Design review of the part built by this model. Coordinates are the model's own, in mm. Coordinates: 2 decimals unless noted, no trailing zeros. Loops run counter-clockwise (first coordinate to the right, second up) from the corner with the lowest first, then second, coordinate; pieces in that order, holes last. Notation, with made-up numbers: (44.5, 56.25) -> (74.5, 56.25) arc R29 ccw to (74.5, 90.25) -> close; hole circle Ø11 at (4.5, 74.25). An arc over 180 degrees is marked (long way). Answer in a Markdown table with one row per item.
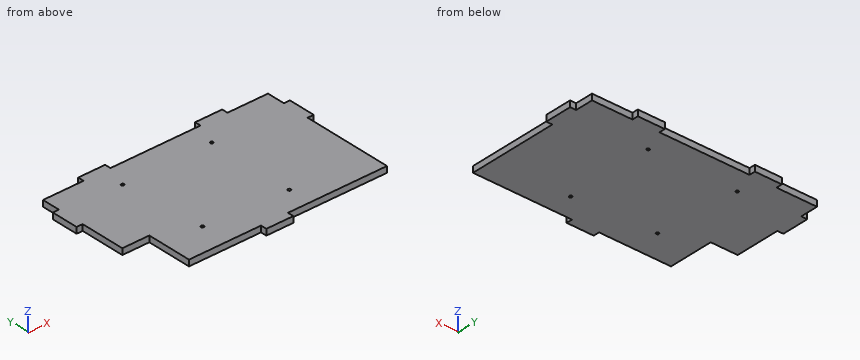
Autodesk Inventor part; units mm, degrees
ref_plane "YZ Plane" through (0, 0, 0) normal (1, 0, 0) x (0, 1, 0)
ref_plane "XZ Plane" through (0, 0, 0) normal (0, 1, 0) x (-1, 0, 0)
ref_plane "XY Plane" through (0, 0, 0) normal (0, 0, 1) x (1, 0, 0)
sketch "Sketch1" plane through (0, 0, 0) normal (0, 0, 1) x (1, 0, 0)
  line L0 (0, 0) -> (250, 0)
  line L1 (250, 0) -> (250, 150)
  line L2 (250, 150) -> (0, 150)
  line L3 (0, 150) -> (0, 0)
  dimension "d0" = 150
  dimension "d1" = 250
extrude "Extrusion1" add sketch "Sketch1" along normal blind 6.731
sketch "Sketch2" plane through (0, 0, 6.731) normal (0, 0, 1) x (1, 0, 0)
  line L0 (0, 0) -> (250, 0)
  line L1 (250, 0) -> (250, 150)
  line L2 (250, 150) -> (0, 150)
  line L3 (0, 150) -> (0, 0)
  point P0 (72.455, 31.185)
  point P1 (65.47, 123.895)
  point P2 (164.53, 123.895)
  point P3 (164.53, 26.105)
  dimension "d4" = 92.075
  dimension "d5" = 5.08
  dimension "d6" = 92.71
  dimension "d7" = 6.985
  dimension "d8" = 26.105
  dimension "d9" = 26.105
  dimension "d10" = 65.47
  dimension "d11" = 85.47
hole "Hole1" at (72.455, 31.185, 6.731) at (65.47, 123.895, 6.731) at (164.53, 123.895, 6.731) at (164.53, 26.105, 6.731) direction (0, 0, -1) diameter 3.176 end through all
sketch "Sketch3" plane through (0, 0, 6.731) normal (0, 0, 1) x (1, 0, 0)
  line L0 (0, 0) -> (250, 0)
  line L1 (250, 0) -> (250, 150)
  line L2 (0, 150) -> (0, 0)
  line L3 (0, 100) -> (-6.731, 100)
  line L4 (-6.731, 100) -> (-6.731, 130)
  line L5 (-6.731, 130) -> (0, 130)
  line L6 (0, 130) -> (0, 100)
  line L7 (250, 130) -> (256.731, 130)
  line L8 (256.731, 130) -> (256.731, 100)
  line L9 (256.731, 100) -> (250, 100)
  line L10 (250, 100) -> (250, 130)
  line L11 (110, 0) -> (140, 0)
  line L12 (140, 0) -> (140, -6.731)
  line L13 (140, -6.731) -> (110, -6.731)
  line L14 (110, -6.731) -> (110, 0)
  line L15 (250, 150) -> (0, 150)
  line L16 (45, 150) -> (75, 150)
  line L17 (75, 150) -> (75, 156.731)
  line L18 (75, 156.731) -> (45, 156.731)
  line L19 (45, 156.731) -> (45, 150)
  line L20 (175, 150) -> (205, 150)
  line L21 (205, 150) -> (205, 156.731)
  line L22 (205, 156.731) -> (175, 156.731)
  line L23 (175, 156.731) -> (175, 150)
  line L24 (75, 156.731) -> (175, 156.731) construction
  point P0 (125, 0)
  point P1 (125, 0)
  point P2 (125, 156.731)
  point P3 (125, 150)
  dimension "d19" = 6.731
  dimension "d20" = 30
  dimension "d21" = 100
  dimension "d24" = 100
extrude "Extrusion2" add sketch "Sketch3" against normal up to surface (6.731 mm away) contours L0 L12 L13 L14 | L3 L4 L5 L2 | L1 L7 L8 L9 | L19 L18 L17 L15 | L23 L22 L21 L15
sketch "Sketch4" plane through (0, 0, 6.731) normal (0, 0, 1) x (1, 0, 0)
  line L0 (0, 0) -> (110, 0)
  line L1 (0, 100) -> (0, 0)
  line L2 (0, 50) -> (30, 50)
  line L3 (30, 50) -> (30, 0)
  dimension "d25" = 50
  dimension "d26" = 30
extrude "Extrusion3" cut sketch "Sketch4" against normal up to next
equation "\"d2\" = THICKB"
equation "\"d19\" = THICKB"
equation "\"THICKA\" = 3.175"
equation "\"THICKB\" = 6.731"
equation "\"THICKC\" = 12.7"
equation "\"THICKPLY\" = 5"
equation "\"MAGDIA\" = 9.5"
equation "\"BALLDIA\" = 12"
properties part number "Center_Mount"
(1) Take a section at B-B on x = 186. Give the boundary of the cut face in (y, z), and give its area (3 significant figures).
Evaluation:
| item | result |
|---|---|
| outline | (0, 0) -> (156.73, 0) -> (156.73, 6.73) -> (0, 6.73) -> close |
| area | 1,050 mm² |
(2) Take a section at C-C on y = 88. Give the boundary of the cut face in (x, z), and give its area (3 significant figures).
Evaluation:
| item | result |
|---|---|
| outline | (0, 0) -> (250, 0) -> (250, 6.73) -> (0, 6.73) -> close |
| area | 1,680 mm² |
(3) For pin 1 (2 mm diameter, centred on x = 252, z = 2, fed in from +Y); pin 2 (2 mm diameter, centred on x = 18, z = 2, fed in from -Y); pin 3 (3.5 mm diameter, centred on x = 53.5, z = 3.5, fed in from -Y); pin 4 (2.5 mm diameter, centred on x = 164.53, y = 123.895, fed in from +Z), all flat-tipped, find the tip position at first contact; note any pin that passes through.
Evaluation:
| item | result |
|---|---|
| pin 1 | stops at y = 130 |
| pin 2 | stops at y = 50 |
| pin 3 | stops at y = 0 |
| pin 4 | passes through |
(4) Take a section at A-A on z = 1.5. Count the separate pieces of the cut face and the enclosed holes in it, and give its area (3 significant figures).
Evaluation:
| item | result |
|---|---|
| separate pieces | 1 |
| enclosed holes | 4 |
| area | 37,000 mm² |
(5) To check wall thickness, follow probe 1 along Y at (x, z) = (164.53, 4); probe 2 along X at (y, z) = (59, 5.5); probe 3 along Y at (x, z) = (143, 3). State the ranges of each line that lie inside material, in increasing order.
Evaluation:
| item | result |
|---|---|
| probe 1 | y = 0 to 24.52, 27.69 to 122.31, 125.48 to 150 |
| probe 2 | x = 0 to 250 |
| probe 3 | y = 0 to 150 |
